```python
from build123d import *

# Parameters (mm, degrees)
SWEEP_1_PROFILE_R   = 11.5
SWEEP_1_PROFILE_R_2 = 9
EXTRUDE_1_DEPTH     = 5
SKETCH_31_R         = 1.7
CUT_EXTRUDE_1_DEPTH = 26
FILLET_1_R          = 0.5
SKETCH_32_R         = 22
SKETCH_32_R_2       = 9
EXTRUDE_5_DEPTH     = 3
EXTRUDE_START       = 3
SKETCH_33_R         = 12
SKETCH_33_R_2       = 9
EXTRUDE_6_DEPTH     = 3
SKETCH_34_R         = 1.7
CUT_EXTRUDE_2_DEPTH = 10


with BuildPart() as part:
    # 扫描-薄件1: sweep along a path in 草图1
    with BuildLine(Plane.XY) as sweep_1_path:
        Line((-40, 27.5), (-27.5, 27.5))
        ThreePointArc((-27.5, 27.5), (-8.054563517, 19.445436483), (0, 0))
    # 扫描-薄件1 profile (on start of the path) → 扫描-薄件1 (sweep)
    with BuildSketch(Plane(origin=(-40, 27.5, 0), x_dir=(0, 1, 0), z_dir=(1, 0, 0))):
        Circle(SWEEP_1_PROFILE_R)
        Circle(SWEEP_1_PROFILE_R_2, mode=Mode.SUBTRACT)
    sweep(path=sweep_1_path.line)

    # 草图30 → 凸台-拉伸1 (add, symmetric)
    with BuildSketch(Plane.ZY.offset(40)):
        with BuildLine():
            ThreePointArc((-10.781929326, 31.5), (-8.76012524, 34.950517149), (-5.678908346, 37.5))
            Line((-5.678908346, 37.5), (-18, 37.5))
            Line((-18, 37.5), (-18, 31.5))
            Line((-18, 31.5), (-10.781929326, 31.5))
        make_face()
        with BuildLine():
            ThreePointArc((-5.678908346, 17.5), (-8.76012524, 20.049482851), (-10.781929326, 23.5))
            Line((-10.781929326, 23.5), (-18, 23.5))
            Line((-18, 23.5), (-18, 17.5))
            Line((-18, 17.5), (-5.678908346, 17.5))
        make_face()
        with BuildLine():
            Line((18, 37.5), (5.678908346, 37.5))
            ThreePointArc((5.678908346, 37.5), (8.76012524, 34.950517149), (10.781929326, 31.5))
            Line((10.781929326, 31.5), (18, 31.5))
            Line((18, 31.5), (18, 37.5))
        make_face()
        with BuildLine():
            Line((18, 17.5), (18, 23.5))
            Line((18, 23.5), (10.781929326, 23.5))
            ThreePointArc((10.781929326, 23.5), (8.76012524, 20.049482851), (5.678908346, 17.5))
            Line((5.678908346, 17.5), (18, 17.5))
        make_face()
    extrude(amount=EXTRUDE_1_DEPTH, both=True)

    # 草图31 → 切除-拉伸1 (cut)
    with BuildSketch(Plane(origin=(0, 37.5, 0), x_dir=(1, 0, 0), z_dir=(0, 1, 0))):
        with Locations(Location((-40, 14, 0), (0, 0, 180))):
            Circle(SKETCH_31_R)
        with Locations(Location((-40, -14, 0), (0, 0, 180))):
            Circle(SKETCH_31_R)
    extrude(amount=-CUT_EXTRUDE_1_DEPTH, mode=Mode.SUBTRACT)

    # 圆角1
    fillet_1_edges = [part.edges().sort_by_distance(p)[0] for p in [
        (-40, 37.5, -18),
        (-45, 34.5, -18),
        (-40, 31.5, -18),
        (-35, 34.5, -18),
        (-40, 31.5, 18),
        (-45, 34.5, 18),
        (-40, 37.5, 18),
        (-35, 34.5, 18),
        (-40, 17.5, 18),
        (-45, 20.5, 18),
        (-40, 23.5, 18),
        (-35, 20.5, 18),
        (-40, 23.5, -18),
        (-45, 20.5, -18),
        (-40, 17.5, -18),
        (-35, 20.5, -18),
        (-42.5, 23.5, 10.781929326),
        (-42.5, 23.5, -10.781929326),
        (-42.5, 31.5, -10.781929326),
        (-42.5, 17.5, 5.678908346),
        (-42.5, 17.5, -5.678908346),
        (-42.5, 37.5, 5.678908346),
        (-42.5, 37.5, -5.678908346),
        (-35, 20.049482851, 8.76012524),
        (-35, 34.950517149, 8.76012524),
        (-35, 20.049482851, -8.76012524),
        (-35, 34.950517149, -8.76012524),
    ]]
    fillet(fillet_1_edges, radius=FILLET_1_R)

    # 草图32 → 凸台-拉伸5 (add)
    with BuildSketch(Plane.XZ):
        Circle(SKETCH_32_R)
        Circle(SKETCH_32_R_2, mode=Mode.SUBTRACT)
    extrude(amount=-EXTRUDE_5_DEPTH)

    # 草图33 → 凸台-拉伸6 (add)
    with BuildSketch(Plane.XZ.offset(EXTRUDE_START)):
        Circle(SKETCH_33_R)
        Circle(SKETCH_33_R_2, mode=Mode.SUBTRACT)
    extrude(amount=-EXTRUDE_6_DEPTH)

    # 草图34 → 切除-拉伸2 (cut)
    with BuildSketch(Plane.XZ):
        with Locations((-12.664726672, 10.981465686)):
            Circle(SKETCH_34_R)
        with Locations((-16.663757776, 1.818534314)):
            Circle(SKETCH_34_R)
        with Locations((16.663757776, -1.818534314)):
            Circle(SKETCH_34_R)
        with Locations((12.664726672, -10.981465686)):
            Circle(SKETCH_34_R)
    extrude(amount=-CUT_EXTRUDE_2_DEPTH, mode=Mode.SUBTRACT)


solid = part.part
```
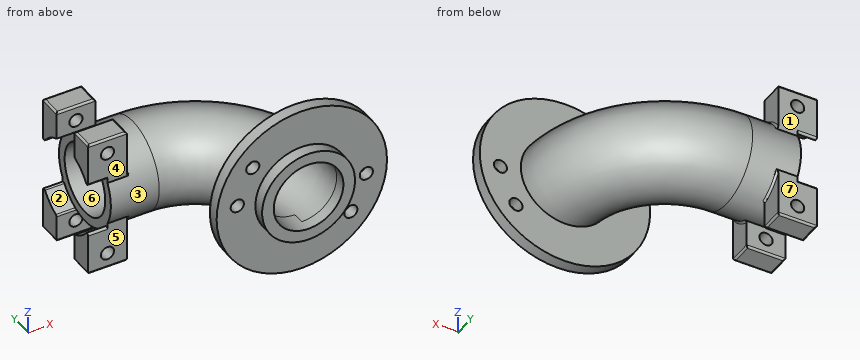
The listing builds one solid part. Answer for the finished solid, in the listing's coordinates (mm). Face numbers are marked on the shaded views. A direction names the side the tool comes from. Give positions to 0.01 mm unless a question says otherwise; leave off trailing zeros. Write each loop counter-clockwise with the first axis right and the second up, starting at its lowest first coordinate (ties: lowest second). Pieces come first, ordered by that corner, then holes. Notation, with made-up numbers: (26.5, 67) -> (64.5, 67) arc R23 ccw to (64.5, 87) -> close; hole circle Ø2 at (-23, 25). An arc over 180 degrees is marked (long way). Write item = value, one per line. Start each with the question number.
1) The part is cut by section B-B, the plane x = -13. Count the separate pieces of the cut face and the enclosed holes in it, and give its area (3 significant figures).
2) The part is cut by section A-A, the plane z = 14. Determine the outline of the cut face in (x, y).
3) Which of the six approach directions +Z, -Z, +X, -X, +Y, -Y give full straight-line access (tool end or side, diameter ignored) to the marked faces 1, 2, 3, 4 and 5?
4) Each of these flat-tipped pins is pushed along its axis until it touches: pin 1 (8.5 mm diameter, centred on x = -41.5, z = 12.5, fed in from +Y); pin 2 (2.5 mm diameter, centred on x = -6.5, z = -3, fed in from +Y); pin 3 (6 mm diameter, centred on x = 10.5, z = 0.5, fed in from +Y). Where does it stop, or does it pass through?
5) Determine the mould class of the marked faces 6 and 7 for opening direction Z: +Z half, -Z half, draft (parallel to the pull), parting line (faces both ways), or undercut.
6) Straight lines are drawn through the part: line 1 along Y through (x, z) = (-15, -2.5); line 2 along Y through (x, z) = (4, -13); line 3 along Y through (x, z) = (-22.5, 2). For each, find the intervals that lie inside material, in ascending order.
Solutions:
q1.separate_pieces = 3
q1.enclosed_holes = 1
q1.area = 306 mm²
q2.outline = (-45, 17.5) -> (-41.7, 17.5) -> (-41.7, 23.5) -> (-45, 23.5) -> close; (-45, 31.5) -> (-41.7, 31.5) -> (-41.7, 37.5) -> (-45, 37.5) -> close; (-38.3, 17.5) -> (-35, 17.5) -> (-35, 23.5) -> (-38.3, 23.5) -> close; (-38.3, 31.5) -> (-35, 31.5) -> (-35, 37.5) -> (-38.3, 37.5) -> close; (-16.97, 0) -> (16.97, 0) -> (16.97, 3) -> (-16.97, 3) -> close
q3.face_1 = +Z, +X, -X, +Y
q3.face_2 = -X
q3.face_3 = none
q3.face_4 = +Z, -X, -Y
q3.face_5 = -Z, -X, -Y
q4.pin_1 = 37.5
q4.pin_2 = 33.25
q4.pin_3 = 17.19
q5.face_6 = undercut
q5.face_7 = draft
q6.line_1 = 0 to 3, 10.42 to 14.11, 33.92 to 36.65
q6.line_2 = 0 to 3
q6.line_3 = 15.38 to 18.05, 35.93 to 38.5
